from build123d import *

# Parameters (mm, degrees)
F0_R     = 3.5
F0_R_2   = 19.05
F1_DEPTH = 11.1125
F2_R     = 5.5
F2_R_2   = 5.4991
F3_DEPTH = 9
F4_R     = 19.05
F5_DEPTH = 10


# Not quite as in the source:
# - a length typed as a fraction of an inch, garbled in the dataset ("3 / 203.2 mm" for 3/8 in), is restored


with BuildPart() as f1:
    # F0 (on Top) → F1 (new body)
    with BuildSketch(Plane.XY):
        Polygon((0, 60), (-60, 60), (-60, -60), (60, -60), (60, 0), (60, 60), align=None)
        with Locations((-45.1685115695, -50.4610737026)):
            Circle(F0_R, mode=Mode.SUBTRACT)
        with Locations((44.6352420051, -50.4610737026)):
            Circle(F0_R, mode=Mode.SUBTRACT)
        with Locations((-45.1685115695, 51.1389262974)):
            Circle(F0_R, mode=Mode.SUBTRACT)
        Circle(F0_R_2, mode=Mode.SUBTRACT)
        with Locations((44.6352420051, 51.1389262974)):
            Circle(F0_R, mode=Mode.SUBTRACT)
    extrude(amount=F1_DEPTH)

    # F2 (on face) → F3 (cut)
    with BuildSketch(Plane.XY.offset(11.1125)):
        with Locations((-45.1685115695, -50.4610737026)):
            Circle(F2_R)
        with Locations((44.6352420051, -50.4610737026)):
            Circle(F2_R_2)
        with Locations((44.6352420051, 51.1389262974)):
            Circle(F2_R_2)
        with Locations((-45.1685115695, 51.1389262974)):
            Circle(F2_R_2)
    extrude(amount=-F3_DEPTH, mode=Mode.SUBTRACT)

    # F4 (on face) → F5 (join)
    with BuildSketch(Plane.XY.offset(11.1125)):
        with BuildLine():
            Line((60, -1.3768154949), (60, 1.3768154949))
            ThreePointArc((60, 1.3768154949), (42.4375754545, 42.4375754545), (1.3768154949, 60))
            Line((1.3768154949, 60), (-1.3768154949, 60))
            ThreePointArc((-1.3768154949, 60), (-42.4375754545, 42.4375754545), (-60, 1.3768154949))
            Line((-60, 1.3768154949), (-60, -1.3768154949))
            ThreePointArc((-60, -1.3768154949), (-42.4375754545, -42.4375754545), (-1.3768154949, -60))
            Line((-1.3768154949, -60), (1.3768154949, -60))
            ThreePointArc((1.3768154949, -60), (42.4375754545, -42.4375754545), (60, -1.3768154949))
        make_face()
        Circle(F4_R, mode=Mode.SUBTRACT)
    extrude(amount=F5_DEPTH)


solid = f1.part
Read the model definition and answer for the solid it produces. Units are mm, in the model's axes. A direction names the side the tool comes from. Round coordinates to 2 decimals unless told otherwise and drop trailing zeros. Write each loop counter-clockwise with the first axis right and the second up, starting at its lowest first coordinate (ties: lowest second). Pieces come first, ordered by that corner, then holes. Notation, with made-up numbers: (79.5, -14.75) - (131.5, -14.75) arc R33 cw to (131.5, 15.25) - close; hole circle Ø10 at (35.25, 53.5). An arc over 180 degrees is marked (long way). Use a Markdown table: item, result.
(1) Straight lines are drawn through the part: line 1 along X through (y, z) = (47.5, 4.5); line 2 along Y through (x, z) = (0, 6.5); line 3 along Y through (x, z) = (-42.5, 2.5). For each, find the intervals that lie inside material, in ascending order. Write a range as [from, to].
Reported:
| item | result |
|---|---|
| line 1 | [-60, -49.29], [-41.05, 40.51], [48.76, 60] |
| line 2 | [-60, -19.05], [19.05, 60] |
| line 3 | [-60, -55.27], [-45.65, 46.33], [55.95, 60] |
(2) Each of these flat-tipped pins is pushed along its axis until it touches: pin 1 Ø5.5 at (x, y) = (-44, -50) entering from +Z; pin 2 Ø5.5 at (x, y) = (-45.17, 51.14) entering from -Z; pin 3 Ø12.5 at (x, y) = (44.64, -50.46) entering from +Z. Where does it stop, or does it pass through?
Reported:
| item | result |
|---|---|
| pin 1 | z = 2.11 |
| pin 2 | through |
| pin 3 | z = 11.11 |
(3) Which of the six approach directions +Z, -Z, +X, -X, +Y, -Y give full straight-line access (tool end or side, diameter ignored) to faces 1 (the cylindrical face through (42.89, 41.98, 16.04)), 2 (the cylindrical face through (-45.88, 56.59, 6.68)), 3 (the flat face through (1, 60, 6)), 4 (the flat face through (47.9, -45.8, 11.112)), 5 (the cylindrical face through (-41.98, 42.89, 16.04))?
Reported:
| item | result |
|---|---|
| face 1 | +Z, +X, +Y |
| face 2 | +Z |
| face 3 | +Z, -Z, +X, -X, +Y |
| face 4 | +Z, +X, -Y |
| face 5 | +Z, -X, +Y |
(4) The part is cut by section C-C (z = 17.5). Write down the section's boundary in (x, y).
Reported:
| item | result |
|---|---|
| outline | (-60, -1.38) arc R60.02 ccw to (-1.38, -60) - (1.38, -60) arc R60.02 ccw to (60, -1.38) - (60, 1.38) arc R60.02 ccw to (1.38, 60) - (-1.38, 60) arc R60.02 ccw to (-60, 1.38) - close; hole circle Ø38.1 at (0, 0) |
(5) The mould has two halves that part along X. Classify faces 6 (the cylindrical face through (-42.89, -41.98, 16.04)), 7 (the cylindrical face through (47.592, 55.776, 6.676)), 8 (the flat face through (-14, 14, 0)): released by +X, released by -X, zero draft, split by the parting line, or undercut.
Reported:
| item | result |
|---|---|
| face 6 | released by -X |
| face 7 | undercut |
| face 8 | zero draft |
(6) The part is cut by section D-D (z = 6.25). Write down the section's boundary in (x, y), then the cut area to 3 significant figures.
Reported:
| item | result |
|---|---|
| outline | (-60, -60) - (60, -60) - (60, 60) - (-60, 60) - close; hole circle Ø11 at (-45.17, -50.46); hole circle Ø11 at (-45.17, 51.14); hole circle Ø38.1 at (0, 0); hole circle Ø11 at (44.64, -50.46); hole circle Ø11 at (44.64, 51.14) |
| area | 12,900 mm2 |
(7) The part is cut by section A-A (x = 0). Write down the section's boundary in (y, z).
Reported:
| item | result |
|---|---|
| outline | (-60, 0) - (-19.05, 0) - (-19.05, 21.11) - (-60, 21.11) - close; (19.05, 0) - (60, 0) - (60, 21.11) - (19.05, 21.11) - close |
